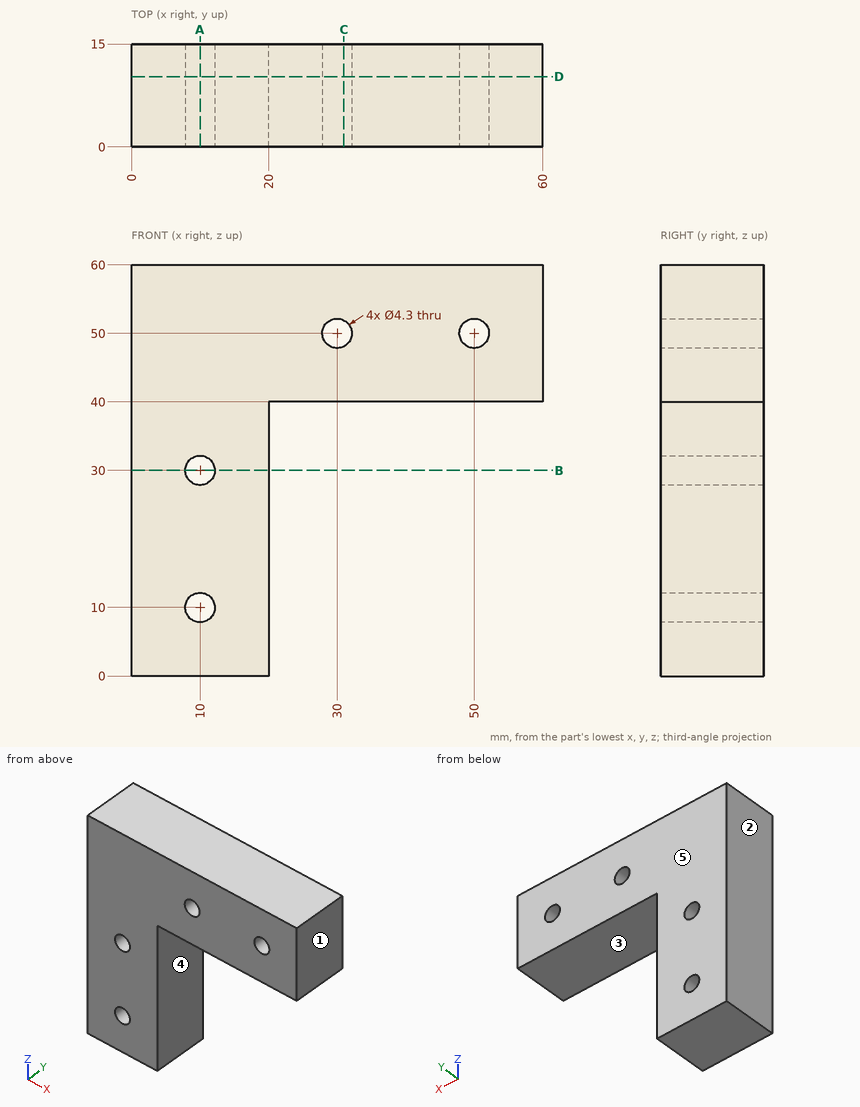
Answer from the drawing. Dimensions are ordinates in mm from the lowest x, y and z of the part. A direction names the side the tool comes from. Give positions to 0.01 mm unless a question says otherwise; leave off trailing zeros. Write each loop counter-clockwise with the first axis right and the second up, starting at its lowest first coordinate (ties: lowest second). Pieces come first, ordered by that corner, then holes. Notation, with made-up numbers: (79, -15.5) - (104, -15.5) arc R16 cw to (104, 1.5) - close; hole circle Ø11 at (78.25, -31.75). An arc over 180 degrees is marked (long way). Answer in a Markdown table with one row per item. Add a question column.
Item 1: Section B-B, the plane z = 30 is taken. Write down the section's boundary in (x, y), and give its area (4 significant figures).
Item 2: Flat-ended cylindrical pins translate along their axes: P1, Ø4.5, axis at x = 38.5, y = 8, coming from the -Z side; P2, Ø1.5, axis at y = 11, z = 9, coming from the +X side; P3, Ø8, axis at y = 9.5, z = 37, coming from the -X side. Find the tip coordinate at first contact, or state that the pin passes through.
Item 3: Section C-C, the plane x = 31 is taken. Write down the section's boundary in (y, z), and give its area (3 significant figures).
Item 4: Find the intervals of material crossed by L1, parallel to X at y = 6.75, z = 50; L2, parallel to X at y = 5, z = 10; L3, parallel to Z at x = 11, y = 1, in increasing order.
Item 5: A tool of negligible diameter and unlimited length cuts with its end or side. For the marked faces 4 and 5, from which of +Z, -Z, +X, -X, +Y, -Y can it reach the whole face along a straight path? Write none if from no direction.
Item 6: Section D-D, the plane y = 10.25 is taken. Write down the section's boundary in (x, z).
Item 7: Section A-A, the plane x = 10 is taken. Write down the section's boundary in (y, z), and give its area (3 significant figures).
Item 8: Determine the mould class of the marked faces 1, 2 and 3 for opening direction X: pulls with the +X half, pulls with the -X half, needs draft (parallel to the pull), parting line crosses it, or undercut.
Recorded:
| question | item | result |
|---|---|---|
| 1 | outline | (0, 0) - (7.85, 0) - (7.85, 15) - (0, 15) - close; (12.15, 0) - (20, 0) - (20, 15) - (12.15, 15) - close |
| 1 | area | 235.5 mm2 |
| 2 | P1 | stops at z = 40 |
| 2 | P2 | stops at x = 20 |
| 2 | P3 | stops at x = 0 |
| 3 | outline | (0, 40) - (15, 40) - (15, 48.1) - (0, 48.1) - close; (0, 51.9) - (15, 51.9) - (15, 60) - (0, 60) - close |
| 3 | area | 243 mm2 |
| 4 | L1 | x = 0 to 27.85, 32.15 to 47.85, 52.15 to 60 |
| 4 | L2 | x = 0 to 7.85, 12.15 to 20 |
| 4 | L3 | z = 0 to 8.1, 11.9 to 28.1, 31.9 to 60 |
| 5 | face 4 | -Z, +X, +Y, -Y |
| 5 | face 5 | +Z, -Z, +X, -X, +Y |
| 6 | outline | (0, 0) - (20, 0) - (20, 40) - (60, 40) - (60, 60) - (0, 60) - close; hole circle Ø4.3 at (10, 10); hole circle Ø4.3 at (10, 30); hole circle Ø4.3 at (30, 50); hole circle Ø4.3 at (50, 50) |
| 7 | outline | (0, 0) - (15, 0) - (15, 7.85) - (0, 7.85) - close; (0, 12.15) - (15, 12.15) - (15, 27.85) - (0, 27.85) - close; (0, 32.15) - (15, 32.15) - (15, 60) - (0, 60) - close |
| 7 | area | 771 mm2 |
| 8 | face 1 | pulls with the +X half |
| 8 | face 2 | pulls with the -X half |
| 8 | face 3 | needs draft |
